Design review of the part shown in the three views and the two pictorial views. Dimensions are in mm from the part's minimum x, y and z. A direction names the side the tool comes from. Give positions to 0.01 mm unless a question says otherwise; leave off trailing zeros. Write each loop counter-clockwise with the first axis right and the second up, starting at its lowest first coordinate (ties: lowest second). Pieces come first, ordered by that corner, then holes. Notation, with made-up numbers: (73.5, 48.25) -> (131.5, 48.25) arc R19 cw to (131.5, 78.25) -> close; hole circle Ø2 at (59, -2). An arc over 180 degrees is marked (long way). Return JSON: item names as keys, results as strings. Group by question number.
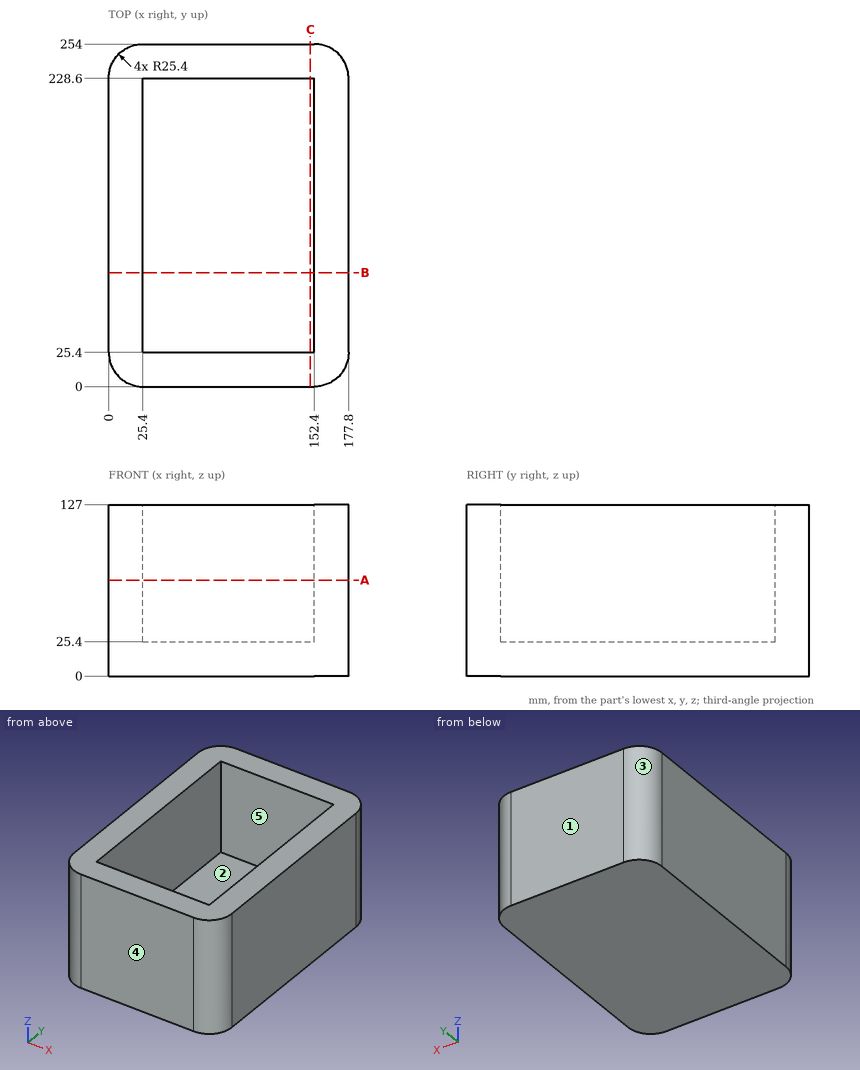
Q1. For L1, parallel to X at y = 78, z = 86; L2, parallel to Y at x = 85, z = 26; L3, parallel to Z at x = 125, y = 50.5, list the stretches that pass through material, from the lowest coordinate up. Write a range as from..to.
Q2. Take a section at B-B, the plane y = 84.5. Give the boundary of the cut face in (x, z).
Q3. Mouldability with a two-part tool opening along Y and no side actions: class the marked faces 3, 4 and 5 as +Y half, -Y half, draft (parallel to the pull), parting line (faces both ways), or undercut.
Q4. Take a section at C-C, the plane x = 149.5. Give the boundary of the cut face in (y, z).
Q5. Take a section at A-A, the plane z = 71. Give the boundary of the cut face in (x, y).
Q6. Tool access review of the marked faces 1 and 2: name each direction out of +Z, -Z, +X, -X, +Y, -Y from which nothing blocks a thin tool from reaching the whole face with its end or side.
Final values:
{
 "1": {"L1": "x = 0..25.4, 152.4..177.8", "L2": "y = 0..25.4, 228.6..254", "L3": "z = 0..25.4"},
 "2": {"outline": "(0, 0) -> (177.8, 0) -> (177.8, 127) -> (152.4, 127) -> (152.4, 25.4) -> (25.4, 25.4) -> (25.4, 127) -> (0, 127) -> close"},
 "3": {"face 3": "+Y half", "face 4": "-Y half", "face 5": "undercut"},
 "4": {"outline": "(0, 0) -> (254, 0) -> (254, 127) -> (228.6, 127) -> (228.6, 25.4) -> (25.4, 25.4) -> (25.4, 127) -> (0, 127) -> close"},
 "5": {"outline": "(0, 25.4) arc R25.4 ccw to (25.4, 0) -> (152.4, 0) arc R25.4 ccw to (177.8, 25.4) -> (177.8, 228.6) arc R25.4 ccw to (152.4, 254) -> (25.4, 254) arc R25.4 ccw to (0, 228.6) -> close; hole (25.4, 25.4) -> (152.4, 25.4) -> (152.4, 228.6) -> (25.4, 228.6) -> close"},
 "6": {"face 1": "+Z, -Z, +X, -X, +Y", "face 2": "+Z"}
}
